Part print with two shaded views. Sizes in mm from the minimum x, y, z corner. Coordinates: 2 decimals unless noted, no trailing zeros. Order: outer loops, then holes, each group sorted by start corner. A loop starts at its lowest first (then second) coordinate and runs counter-clockwise, first axis right, second up. Notation, with made-up numbers: (-26.5, -18.5) - (-5.5, -18.5) arc R25 cw to (-5.5, 16.5) - close; hole circle Ø9 at (43, -24). An arc over 180 degrees is marked (long way). Return JSON: item names as keys, results as strings.
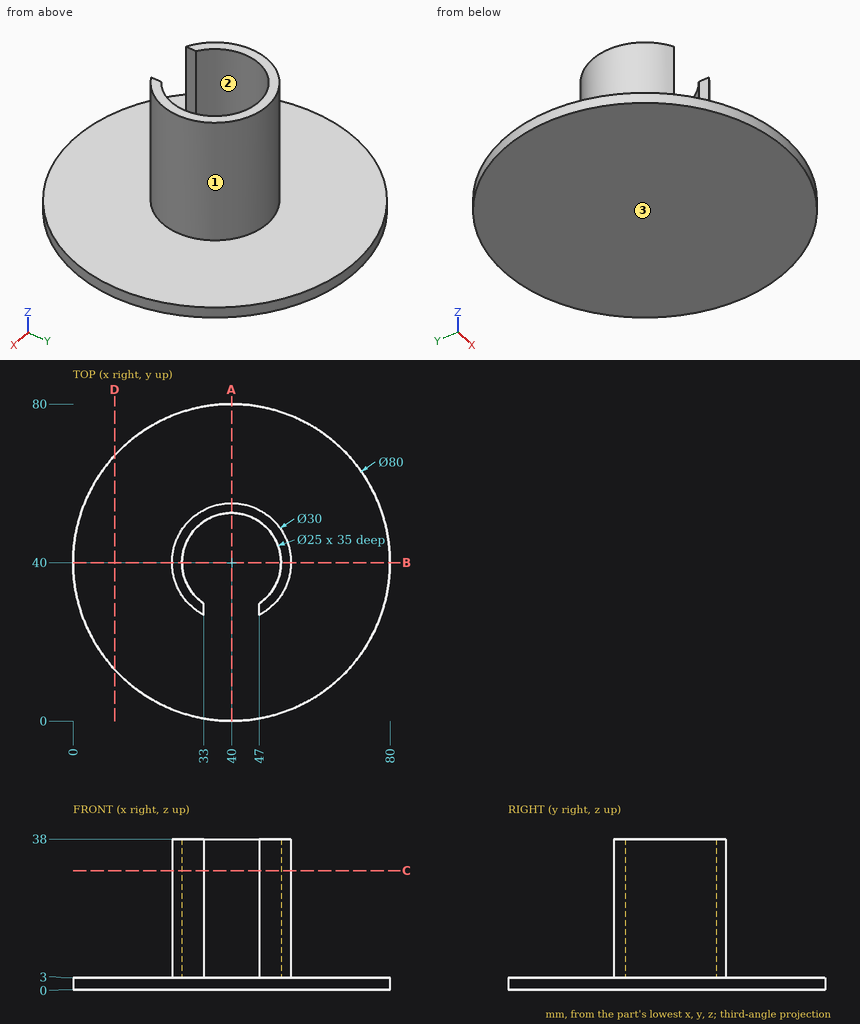
Item 1: Band-saw the part on D-D, the plane x = 10.5. List the corners of the cut face in (y, z).
Findings below:
{"outline": "(12.99, 0) - (67.01, 0) - (67.01, 3) - (12.99, 3) - close"}
Item 2: Mould opens along Y. For the marked faces 1, 2 and 3 say: released by +Y, released by -Y, zero draft, split by the parting line, or undercut.
Findings below:
{"face 1": "split by the parting line", "face 2": "undercut", "face 3": "zero draft"}
Item 3: Band-saw the part on C-C, the plane z = 30. List the corners of the cut face in (x, y), then the cut area to 3 significant figures.
Findings below:
{"outline": "(33, 26.73) - (33, 29.64) arc R12.5 cw (long way) to (47, 29.64) - (47, 26.73) arc R15 ccw (long way) to start", "area": "179 mm²"}
Item 4: Wall check: L1, parallel to X at y = 40, z = 20; L2, parallel to Z at x = 38.5, y = 8; L3, parallel to Y at x = 35, z = 32. Give the ranges that are in metal, low to high. Write a range as [from, to].
Findings below:
{"L1": "x = [25, 27.5], [52.5, 55]", "L2": "z = [0, 3]", "L3": "y = [51.46, 54.14]"}
Item 5: Band-saw the part on A-A, the plane x = 40. List the corners of the cut face in (y, z).
Findings below:
{"outline": "(0, 0) - (80, 0) - (80, 3) - (55, 3) - (55, 38) - (52.5, 38) - (52.5, 3) - (0, 3) - close"}
Item 6: Drop flat-ended pins along their axis: P1, Ø1.5, axis at y = 46.5, z = 11, coming from the +X side; P2, Ø1.5, axis at y = 28.5, z = 21, coming from the -X side; P3, Ø8, axis at x = 40.5, y = 22.5, coming from the +Z side. Give the stop position or say it passes through.
Findings below:
{"P1": "stops at x = 53.85", "P2": "stops at x = 29.54", "P3": "stops at z = 3"}
Item 7: Band-saw the part on B-B, the plane y = 40. List the corners of the cut face in (x, z).
Findings below:
{"outline": "(0, 0) - (80, 0) - (80, 3) - (55, 3) - (55, 38) - (52.5, 38) - (52.5, 3) - (27.5, 3) - (27.5, 38) - (25, 38) - (25, 3) - (0, 3) - close"}
